```python
from build123d import *

# Parameters (mm, degrees)
BOSS_EXTRUDE1_DEPTH = 50
SHELL1_DEPTH        = 50
CUT_EXTRUDE2_DEPTH  = 173.364622498


# Read off the part's stored shape, not the designer's step: Shell1
with BuildPart() as part:
    # Sketch1 → Boss-Extrude1 (new body)
    with BuildSketch(Plane.YZ):
        with BuildLine():
            Line((-44.627499653, -40.034766679), (-44.627499653, 40.034766679))
            Line((-44.627499653, 40.034766679), (-29.010308673, 78.667639283))
            ThreePointArc((-29.010308673, 78.667639283), (-28.186204205, 80.272180413), (-27.087258828, 81.702571783))
            Line((-27.087258828, 81.702571783), (-3.674040134, 107.06723584))
            ThreePointArc((-3.674040134, 107.06723584), (0, 108.675860147), (3.674040134, 107.06723584))
            Line((3.674040134, 107.06723584), (27.087258828, 81.702571783))
            ThreePointArc((27.087258828, 81.702571783), (28.186204205, 80.272180413), (29.010308673, 78.667639283))
            Line((29.010308673, 78.667639283), (44.627499653, 40.034766679))
            Line((44.627499653, 40.034766679), (44.627499653, -40.034766679))
            Line((44.627499653, -40.034766679), (0, -138.719530665))
            Line((0, -138.719530665), (-44.627499653, -40.034766679))
        make_face()
    extrude(amount=BOSS_EXTRUDE1_DEPTH)

    # Shell1 outline → Shell1 (cut)
    with BuildSketch(Plane.YZ):
        with BuildLine():
            Line((-24.374743616, 76.79372984), (-39.627499653, 39.062374592))
            Line((-39.627499653, 39.062374592), (-39.627499653, -38.956762217))
            Line((-39.627499653, -38.956762217), (0, -126.585029116))
            Line((0, -126.585029116), (39.627499653, -38.956762217))
            Line((39.627499653, -38.956762217), (39.627499653, 39.062374592))
            Line((39.627499653, 39.062374592), (24.374743616, 76.79372984))
            ThreePointArc((24.374743616, 76.79372984), (23.962691382, 77.596000405), (23.413218693, 78.31119609))
            Line((23.413218693, 78.31119609), (0, 103.675860147))
            Line((0, 103.675860147), (-23.413218693, 78.31119609))
            ThreePointArc((-23.413218693, 78.31119609), (-23.962691382, 77.596000405), (-24.374743616, 76.79372984))
        make_face()
    extrude(amount=SHELL1_DEPTH, mode=Mode.SUBTRACT)

    # Sketch3 → Cut-Extrude2 (cut, through all)
    with BuildSketch(Plane(origin=(0, 44.627499653, 0), x_dir=(-1, 0, 0), z_dir=(0, 1, 0))):
        Polygon((-50, -40.034766679), (-25, -138.719530665), (-50, -138.719530665), align=None)
    extrude(amount=-CUT_EXTRUDE2_DEPTH, mode=Mode.SUBTRACT)


solid = part.part
```
Geometry check sheet. Reference: the model listing, model coordinates, mm. A direction names the side the tool comes from. Coordinates: 2 decimals unless noted, no trailing zeros. Order: outer loops, then holes, each group sorted by start corner. A loop starts at its lowest first (then second) coordinate and runs counter-clockwise, first axis right, second up. Notation, with made-up numbers: M 11,7.25 L 30,7.25 A24 ccw 30,37.25 Z; hole C -16.5,40 d9. An arc over 180 degrees is marked long. One line per question, with ' | ' between items. Start each with the question number.
Item 1: Cross-section at C-C on y = -10. Enter the section's corners in (x, z), then the cut area to 3 significant figures.
Item 2: Material ranges on L1, parallel to Y at x = 41, z = -5; L2, parallel to Y at x = 37.5, z = 81.5; L3, parallel to Z at x = 23, y = 35, recorded low to high. Write a range as [from, to].
Item 3: Draft check along Z on faces 1 (the flat face through (24.65, 36.71, 59.62)), 2 (the flat face through (19.09, -20.09, -82.16)), 3 (the flat face through (36.632, -16.32, -92.802)). Enter one of: pulls with the +Z half, pulls with the -Z half, needs draft (parallel to the pull), parting line crosses it, or undercut.
Item 4: Cross-section at A-A on x = 9.5. Enter the section's corners in (y, z), then the cut area to 3 significant figures.
Item 5: Cross-section at D-D on x = 35.5. Enter the section's corners in (y, z), then the cut area to 3 significant figures.
Item 6: Set-up check for faces 4 (the flat face through (25, 44.627, 1)), 5 (the flat face through (25, -39.627, 1)): record each of +Z, -Z, +X, -X, +Y, -Y from which the full face is reachable in a straight line by a thin tool's end or side.
Item 7: Gauge pin test, flat ends, axial feed: pin 1 (5 mm diameter, centred on x = 13.5, z = 76, fed in from +Y); pin 2 (12 mm diameter, centred on x = 7.5, z = 44, fed in from -Y); pin 3 (3 mm diameter, centred on x = 18, y = 16, fed in from +Z); pin 4 (10 mm diameter, centred on x = 14, y = -20, fed in from -Z). Record the tip position at first contact, or that the pin passes through.
Item 8: Cross-section at B-B on z = -103.5. Enter the section's corners in (x, y).
Findings:
1) outline: M 0,-116.61 L 30.6,-116.61 L 33.68,-104.47 L 0,-104.47 Z; M 0,92.84 L 50,92.84 L 50,100.21 L 0,100.21 Z | area: 759 mm²
2) L1: y = [-44.63, -39.63], [39.63, 44.63] | L2: y = [-27.27, -20.47], [20.47, 27.27] | L3: z = [-61.32, -49.19], [50.51, 63.85]
3) face 1: pulls with the +Z half | face 2: undercut | face 3: pulls with the -Z half
4) outline: M -44.63,-40.03 L 0,-138.72 L 44.63,-40.03 L 44.63,40.03 L 29.01,78.67 A10 ccw 27.09,81.7 L 3.67,107.07 A5 ccw -3.67,107.07 L -27.09,81.7 A10 ccw -29.01,78.67 L -44.63,40.03 Z; hole M -39.63,-38.96 L 0,-126.59 L 39.63,-38.96 L 39.63,39.06 L 24.37,76.79 A5 ccw 23.41,78.31 L 0,103.68 L -23.41,78.31 A5 ccw -24.37,76.79 L -39.63,39.06 Z | area: 2,620 mm²
5) outline: M -44.63,-40.03 L -18.74,-97.27 L -13.26,-97.27 L -39.63,-38.96 L -39.63,39.06 L -24.37,76.79 A5 cw -23.41,78.31 L 0,103.68 L 23.41,78.31 A5 cw 24.37,76.79 L 39.63,39.06 L 39.63,-38.96 L 13.26,-97.27 L 18.74,-97.27 L 44.63,-40.03 L 44.63,40.03 L 29.01,78.67 A10 ccw 27.09,81.7 L 3.67,107.07 A5 ccw -3.67,107.07 L -27.09,81.7 A10 ccw -29.01,78.67 L -44.63,40.03 Z | area: 2,230 mm²
6) face 4: +Z, -Z, +X, -X, +Y | face 5: +X, -X
7) pin 1: stops at y = 31.1 | pin 2: stops at y = -44.63 | pin 3: stops at z = 95.34 | pin 4: stops at z = -105.55
8) outline: M 0,-15.93 L 33.92,-15.93 L 33.92,-10.44 L 0,-10.44 Z; M 0,10.44 L 33.92,10.44 L 33.92,15.93 L 0,15.93 Z
